CAD build for the part. Positions are in the model's coordinates, mm. Round coordinates to 2 decimals unless told otherwise and drop trailing zeros. Order: outer loops, then holes, each group sorted by start corner. A loop starts at its lowest first (then second) coordinate and runs counter-clockwise, first axis right, second up. Notation, with made-up numbers: M 87,30.25 L 112,30.25 A8 ccw 112,38.25 Z; hole C -27.5,-4.5 d11. An arc over 180 degrees is marked long. Put each result on its own line as item: value.
```python
from build123d import *

# Parameters (mm, degrees)
SKETCH_1_W          = 125
SKETCH_1_H          = 65
EXTRUDE_1_DEPTH     = 3
SKETCH_2_R          = 1.55
SKETCH_2_R_2        = 2.1
SKETCH_2_R_3        = 7.5
CUT_EXTRUDE_1_DEPTH = 3
FILLET_1_R          = 5


with BuildPart() as part:
    # 草图1 → 凸台-拉伸1 (new body)
    with BuildSketch(Plane(origin=(0, 0, 0), x_dir=(1, 0, 0), z_dir=(0, 1, 0))):
        Rectangle(SKETCH_1_W, SKETCH_1_H)
    extrude(amount=EXTRUDE_1_DEPTH)

    # 草图2 → 切除-拉伸1 (cut)
    with BuildSketch(Plane(origin=(0, 0, 0), x_dir=(-1, 0, 0), z_dir=(0, -1, 0))):
        with Locations(Location((-50, 22.5, 0), (0, 0, 90))):
            Circle(SKETCH_2_R)
        with Locations(Location((-50, -25.5, 0), (0, 0, 90))):
            Circle(SKETCH_2_R)
        with Locations(Location((50, 22.5, 0), (0, 0, 90))):
            Circle(SKETCH_2_R)
        with Locations(Location((50, -25.5, 0), (0, 0, 90))):
            Circle(SKETCH_2_R)
        with Locations(Location((-14.5, -23.480762114, 0), (0, 0, 90))):
            Circle(SKETCH_2_R_2)
        with Locations(Location((-14.5, 28.480762114, 0), (0, 0, 90))):
            Circle(SKETCH_2_R_2)
        with Locations(Location((30.5, 2.5, 0), (0, 0, 90))):
            Circle(SKETCH_2_R_2)
        with Locations(Location((0.5, 2.5, 0), (0, 0, 90))):
            Circle(SKETCH_2_R_3)
    extrude(amount=-CUT_EXTRUDE_1_DEPTH, mode=Mode.SUBTRACT)

    # 圆角1
    fillet_1_edges = [part.edges().sort_by_distance(p)[0] for p in [
        (62.5, 1.5, 32.5),
        (-62.5, 1.5, 32.5),
        (-62.5, 1.5, -32.5),
        (62.5, 1.5, -32.5),
    ]]
    fillet(fillet_1_edges, radius=FILLET_1_R)


solid = part.part
```
Item 1: Band-saw the part on D-D on x = -50. Give the cut face in (y, z), and give its area (3 significant figures).
Answers below:
outline: M 0,-32.5 L 3,-32.5 L 3,-24.05 L 0,-24.05 Z; M 0,-20.95 L 3,-20.95 L 3,23.95 L 0,23.95 Z; M 0,27.05 L 3,27.05 L 3,32.5 L 0,32.5 Z
area: 176 mm²
Item 2: Band-saw the part on C-C on x = -30.5. Give the cut face in (y, z).
Answers below:
outline: M 0,-32.5 L 3,-32.5 L 3,-4.6 L 0,-4.6 Z; M 0,-0.4 L 3,-0.4 L 3,32.5 L 0,32.5 Z
Item 3: Band-saw the part on B-B on y = 1.6. State how many separate pieces and enclosed holes the cut face has, and give its area (3 significant figures).
Answers below:
separate pieces: 1
enclosed holes: 8
area: 7,860 mm²
Item 4: Band-saw the part on A-A on z = -2.5. Give the cut face in (x, y), and give its area (3 significant figures).
Answers below:
outline: M -62.5,0 L -32.6,0 L -32.6,3 L -62.5,3 Z; M -28.4,0 L -8,0 L -8,3 L -28.4,3 Z; M 7,0 L 62.5,0 L 62.5,3 L 7,3 Z
area: 317 mm²
Item 5: Probe line 1 along X through (y, z) = (1.75, -2.5); line 2 along X through (y, z) = (1.3, -22.5); line 3 along X through (y, z) = (2.85, 24.5). List the from-to ranges inside material, lowest first. Write a range as [from, to].
Answers below:
line 1: [-62.5, -32.6], [-28.4, -8], [7, 62.5]
line 2: [-62.5, -51.55], [-48.45, 48.45], [51.55, 62.5]
line 3: [-62.5, -51.18], [-48.82, 12.66], [16.34, 48.82], [51.18, 62.5]
Item 6: Mould opens along X. For faces 1 (the flat face through (-1, 3, 7)), 2 (the flat face through (62.5, 1, 0)), 3 (the cylindrical face through (48.487, 1.479, 25.836)) say: pulls with the +X half, pulls with the -X half, needs draft (parallel to the pull), parting line crosses it, or undercut.
Answers below:
face 1: needs draft
face 2: pulls with the +X half
face 3: undercut
